```python
from build123d import *

# Parameters (mm, degrees)
SKETCH1_R           = 2.5
BOSS_EXTRUDE1_DEPTH = 10
SKETCH2_W           = 10
SKETCH2_H           = 15
SKETCH2_R           = 2.5
SKETCH2_H_2         = 10.4
BOSS_EXTRUDE2_DEPTH = 5
FILLET1_R           = 5
FILLET2_R           = 1.5
FILLET3_R           = 1


with BuildPart() as part:
    # Sketch1 → Boss-Extrude1 (new body)
    with BuildSketch(Plane.XY):
        with BuildLine():
            Line((-5, 0), (-5, -12))
            Line((-5, -12), (5, -12))
            Line((5, -12), (5, 0))
            ThreePointArc((5, 0), (0, 5), (-5, 0))
        make_face()
        Circle(SKETCH1_R, mode=Mode.SUBTRACT)
    extrude(amount=BOSS_EXTRUDE1_DEPTH)

    # Sketch2 → Boss-Extrude2 (add)
    # profile 1 of 2: a face of its own
    with BuildSketch(Plane.XZ.offset(12)):
        with Locations((0, -7.5)):
            Rectangle(SKETCH2_W, SKETCH2_H)
        with Locations(Location((0, -10, 0), (0, 0, 270))):
            Circle(SKETCH2_R, mode=Mode.SUBTRACT)
    # profile 2 of 2: a face of its own
    with BuildSketch(Plane.XZ.offset(12)):
        with Locations((0, 15.2)):
            Rectangle(SKETCH2_W, SKETCH2_H_2)
        with Locations(Location((0, 15.4, 0), (0, 0, 270))):
            Circle(SKETCH2_R, mode=Mode.SUBTRACT)
    extrude(amount=-BOSS_EXTRUDE2_DEPTH)

    # Fillet1
    fillet1_edges = [part.edges().sort_by_distance(p)[0] for p in [
        (5, -9.5, -15),
        (5, -9.5, 20.4),
        (-5, -9.5, 20.4),
        (-5, -9.5, -15),
    ]]
    fillet(fillet1_edges, radius=FILLET1_R - 0.0001)  # a hair under: the kernel refuses the full size

    # Fillet2
    fillet2_edges = [part.edges().sort_by_distance(p)[0] for p in [
        (0, -7, 0),
        (0, -7, 10),
    ]]
    fillet(fillet2_edges, radius=FILLET2_R)

    # Fillet3
    fillet3_edges = [part.edges().sort_by_distance(p)[0] for p in [
        (5, -2.75, 10),
        (0, 5, 10),
        (-5, -2.75, 10),
        (-5, -12, 2.7),
        (5, -12, 2.7),
        (-3.535563195, -12, -13.535563195),
        (3.535563195, -12, -13.535563195),
        (-3.535563195, -12, 18.935563195),
        (3.535563195, -12, 18.935563195),
        (5, -7, -5.75005),
        (-3.535563195, -7, -13.535563195),
        (3.535563195, -7, -13.535563195),
        (-5, -7, 13.45005),
        (-3.535563195, -7, 18.935563195),
        (3.535563195, -7, 18.935563195),
        (5, -7, 13.45005),
        (-5, -7, -5.75005),
        (5, -6.560660172, 10.439339828),
        (-5, -6.560660172, 10.439339828),
        (-5, -6.560660172, -0.439339828),
        (5, -6.560660172, -0.439339828),
        (-5, -2.75, 0),
        (0, 5, 0),
        (5, -2.75, 0),
    ]]
    fillet(fillet3_edges, radius=FILLET3_R)


solid = part.part
```
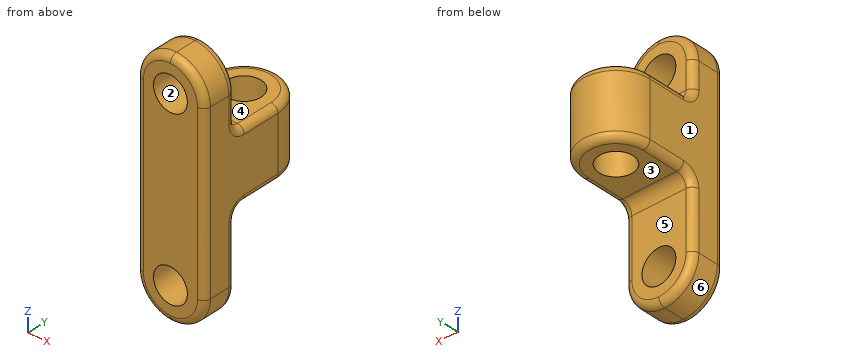
Here's how the part is built. I have some questions about the finished solid (model axes, mm). Face numbers are marked on the shaded views. A direction names the side the tool comes from. Give positions to 0.01 mm unless a question says otherwise; leave off trailing zeros. Write each loop counter-clockwise with the first axis right and the second up, starting at its lowest first coordinate (ties: lowest second). Pieces come first, ordered by that corner, then holes. Notation, with made-up numbers: (-2.5, 83) -> (5.5, 83) arc R10 ccw to (5.5, 96) -> close; hole circle Ø10 at (76, -3.75). An arc over 180 degrees is marked (long way). Write each question's results on one line, items separated by ' | '.
Item 1: On a 3-axis mill with a long thin cutter (end or side, diameter ignored), from which of +Z, -Z, +X, -X, +Y, -Y can I reach the whole of each face in a straight line? I mean the marked faces 4, 5 and 6. Say none if no direction works.
Output:
face 4: +Z, +X, -X, +Y | face 5: -Z, +X, -X, +Y | face 6: -Z, -X, +Y, -Y
Item 2: If I drill on L1, parallel to Y at x = 0, z = 7.5; L2, parallel to X at y = -10.2, z = -10; L3, parallel to Y at x = -1.5, z = 3, over which ranges is the centre line in solid material (lowest first)?
Output:
L1: y = -12 to -2.5, 2.5 to 5 | L2: x = -5 to -2.5, 2.5 to 5 | L3: y = -12 to -2, 2 to 4.77
Item 3: Suppose I cut it at A-A on y = -2. Write out the boundary of the cut face in (x, z).
Output:
outline: (-5, 1) arc R1 ccw to (-4, 0) -> (-1.5, 0) -> (-1.5, 10) -> (-4, 10) arc R1 ccw to (-5, 9) -> close; (1.5, 0) -> (4, 0) arc R1 ccw to (5, 1) -> (5, 9) arc R1 ccw to (4, 10) -> (1.5, 10) -> close
Item 4: Suppose I cut it at B-B on z = -9. Write out the boundary of the cut face in (x, y).
Output:
outline: (-5, -11) arc R1 ccw to (-4, -12) -> (-2.29, -12) -> (-2.29, -7) -> (-4, -7) arc R1 ccw to (-5, -8) -> close; (2.29, -12) -> (4, -12) arc R1 ccw to (5, -11) -> (5, -8) arc R1 ccw to (4, -7) -> (2.29, -7) -> close
Item 5: Suppose I cut it at C-C on z = -4.5. Write out the boundary of the cut face in (x, y), plus the area to 3 significant figures.
Output:
outline: (-5, -11) arc R1 ccw to (-4, -12) -> (4, -12) arc R1 ccw to (5, -11) -> (5, -8) arc R1 ccw to (4, -7) -> (-4, -7) arc R1 ccw to (-5, -8) -> close | area: 49.1 mm^2
Item 6: Suppose I cut it at D-D on y = -4.25. Write out the boundary of the cut face in (x, z).
Output:
outline: (-5, 1) arc R1 ccw to (-4, 0) -> (4, 0) arc R1 ccw to (5, 1) -> (5, 9) arc R1 ccw to (4, 10) -> (-4, 10) arc R1 ccw to (-5, 9) -> close
Item 7: We'd pull the mould along Z, two halves only. Please class the marked faces 1, 2 and 3: pulls with the +Z half, pulls with the -Z half, needs draft (parallel to the pull), parting line crosses it, or undercut.
Output:
face 1: needs draft | face 2: undercut | face 3: pulls with the -Z half
Item 8: For pin 1 Ø2.5 at (x, y) = (-2, -3) entering from -Z; pin 2 Ø2.5 at (x, y) = (2, -1.5) entering from +Z; pin 3 Ø2.5 at (x, z) = (0, 15.5) entering from +Y, each with a flat end and sliding along its axis, tell me the tip position at first contact or that it passes through.
Output:
pin 1: stops at z = 0 | pin 2: stops at z = 10 | pin 3: passes through
